Study the drawing (mm; zero at the part's minimum x, y, z) and answer. A direction names the side the tool comes from. Round coordinates to 2 decimals unless told otherwise and drop trailing zeros. Write each loop counter-clockwise with the first axis right and the second up, starting at its lowest first coordinate (ties: lowest second). Pieces come first, ordered by that corner, then holes. Notation, with made-up numbers: (67, -19.75) -> (119, -19.75) arc R29 cw to (119, 2.25) -> close; hole circle Ø1 at (-8.75, 74.5). An arc over 180 degrees is marked (long way). Return JSON: item names as keys, results as strings.
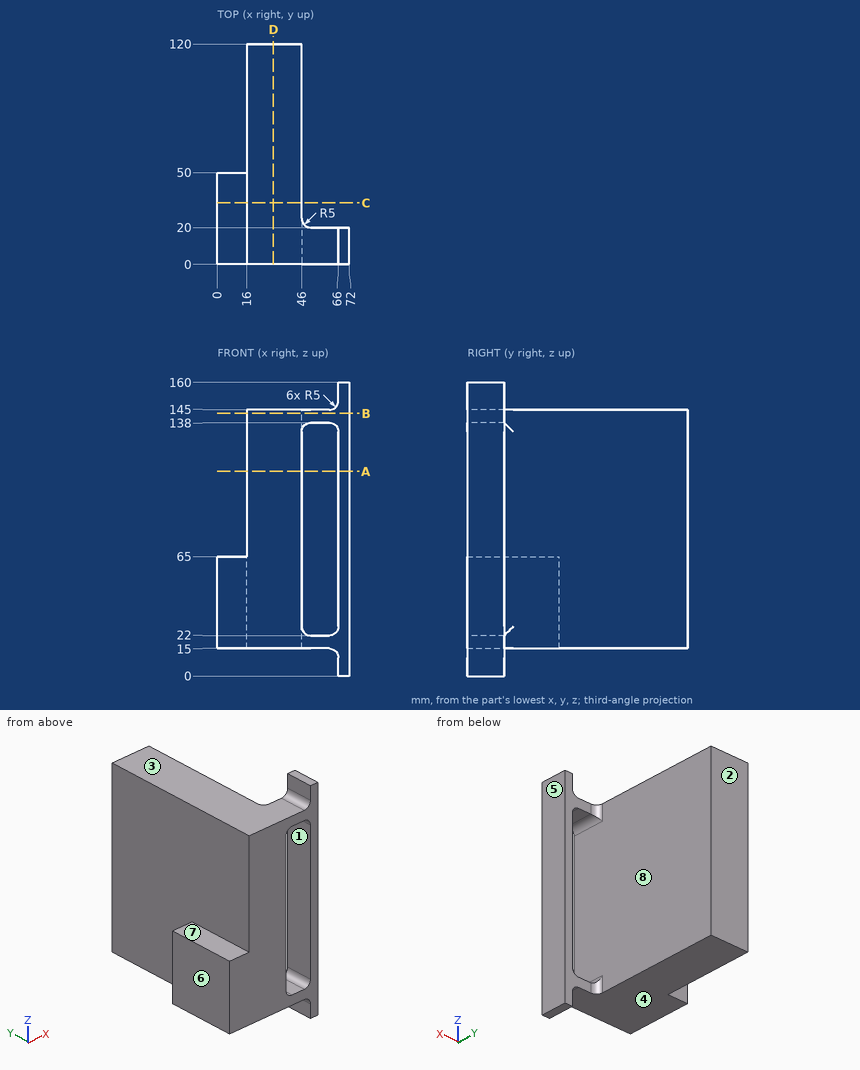
Item 1: A tool of negligible diameter and unlimited length cuts with its end or side. For the marked faces 1, 2, 3 and 4, from which of +Z, -Z, +X, -X, +Y, -Y can it reach the whole face along a straight path? Write none if from no direction.
Worked answers:
{"face 1": "+Y, -Y", "face 2": "+Z, -Z, +X, -X, +Y", "face 3": "+Z, -X, +Y, -Y", "face 4": "-Z, -X, +Y, -Y"}
Item 2: Section D-D (x = 30.5) is taken. Give the vertices of the cut face in (y, z), then the cut area to 3 significant figures.
Worked answers:
{"outline": "(0, 15) -> (120, 15) -> (120, 145) -> (0, 145) -> close", "area": "15,600 mm2"}
Item 3: Section B-B (z = 143) is taken. Give the vertices of the cut face in (x, y), then the cut area to 3 significant figures.
Worked answers:
{"outline": "(16, 0) -> (72, 0) -> (72, 20) -> (51, 20) arc R5 cw to (46, 25) -> (46, 120) -> (16, 120) -> close", "area": "4,130 mm2"}
Item 4: Section C-C (y = 33.5) is taken. Give the vertices of the cut face in (x, z).
Worked answers:
{"outline": "(0, 15) -> (46, 15) -> (46, 145) -> (16, 145) -> (16, 65) -> (0, 65) -> close"}
Item 5: Straight lines are drawn through the part: L1, parallel to Z at x = 55, y = 18; L2, parallel to X at y = 30.5, z = 68.5; L3, parallel to Z at x = 43, y = 6. For each, find the intervals that lie inside material, in ascending order. Write a range as [from, to].
Worked answers:
{"L1": "z = [15, 22], [138, 145]", "L2": "x = [16, 46]", "L3": "z = [15, 145]"}
Item 6: Flat-ended cylindrical pins translate along their axes: pin 1 (22.5 mm diameter, centred on x = 28.5, y = 63, fed in from +Z); pin 2 (5 mm diameter, centred on y = 55, z = 65.5, fed in from -X); pin 3 (8 mm diameter, centred on y = 5, z = 6, fed in from -X); pin 4 (1 mm diameter, centred on x = 20, z = 20, fed in from -Y). Find the tip coordinate at first contact, or state that the pin passes through.
Worked answers:
{"pin 1": "stops at z = 145", "pin 2": "stops at x = 16", "pin 3": "stops at x = 66", "pin 4": "stops at y = 0"}
Item 7: Section A-A (z = 111.5) is taken. Give the vertices of the cut face in (x, y), then the cut area to 3 significant figures.
Worked answers:
{"outline": "(16, 0) -> (46, 0) -> (46, 120) -> (16, 120) -> close; (66, 0) -> (72, 0) -> (72, 20) -> (66, 20) -> close", "area": "3,720 mm2"}
Item 8: For a pull along X with two mould halves and no side action, classify the marked faces 5, 6, 7 and 8 as released by +X, released by -X, zero draft, split by the parting line, or undercut.
Worked answers:
{"face 5": "released by +X", "face 6": "released by -X", "face 7": "zero draft", "face 8": "undercut"}
